CAD build for the part. Positions are in the model's coordinates, mm. A direction names the side the tool comes from. Give positions to 0.01 mm unless a question says otherwise; leave off trailing zeros. Loops run counter-clockwise (first coordinate to the right, second up) from the corner with the lowest first, then second, coordinate; pieces in that order, holes last. Notation, with made-up numbers: M -34.75,76 L -26.75,76 A25 cw -26.75,115 Z; hole C 51.25,25 d4. An arc over 180 degrees is marked long. One line per question, with ' | ' between items.
```python
from build123d import *

# Parameters (mm, degrees)
BOSS_EXTRUDE1_DEPTH      = 1.5
M3_CLEARANCE_HOLE1_D     = 3.2
M3_CLEARANCE_HOLE1_DEPTH = 3
SKETCH5_R                = 15
CUT_EXTRUDE1_DEPTH       = 1
CUT_EXTRUDE1_DEPTH_BACK  = 4
SKETCH6_R                = 13
BOSS_EXTRUDE2_DEPTH      = 40
M6_CLEARANCE_HOLE1_D     = 6.4
M6_CLEARANCE_HOLE1_DEPTH = 10
SKETCH11_OUTSIDE_W       = 233.632
SKETCH11_OUTSIDE_H       = 233.632
CUT_EXTRUDE2_DEPTH       = 40
SKETCH12_W               = 183.089507272
SKETCH12_H               = 5.144734847
CUT_EXTRUDE4_DEPTH       = 91
CUT_EXTRUDE4_DEPTH_BACK  = 91


with BuildPart() as part:
    # Sketch1 → Boss-Extrude1 (new body, symmetric)
    with BuildSketch(Plane(origin=(0, 0, 0), x_dir=(1, 0, 0), z_dir=(0, 1, 0))):
        with BuildLine():
            Line((50, 10), (84, 10))
            ThreePointArc((84, 10), (88.242640687, 8.242640687), (90, 4))
            Line((90, 4), (90, -4))
            ThreePointArc((90, -4), (88.242640687, -8.242640687), (84, -10))
            Line((84, -10), (50, -10))
            ThreePointArc((50, -10), (21.715728753, -21.715728753), (10, -50))
            Line((10, -50), (10, -84))
            ThreePointArc((10, -84), (8.242640687, -88.242640687), (4, -90))
            Line((4, -90), (-4, -90))
            ThreePointArc((-4, -90), (-8.242640687, -88.242640687), (-10, -84))
            Line((-10, -84), (-10, -50))
            ThreePointArc((-10, -50), (-21.715728753, -21.715728753), (-50, -10))
            Line((-50, -10), (-84, -10))
            ThreePointArc((-84, -10), (-88.242640687, -8.242640687), (-90, -4))
            Line((-90, -4), (-90, 4))
            ThreePointArc((-90, 4), (-88.242640687, 8.242640687), (-84, 10))
            Line((-84, 10), (-50, 10))
            ThreePointArc((-50, 10), (-21.715728753, 21.715728753), (-10, 50))
            Line((-10, 50), (-10, 84))
            ThreePointArc((-10, 84), (-8.242640687, 88.242640687), (-4, 90))
            Line((-4, 90), (4, 90))
            ThreePointArc((4, 90), (8.242640687, 88.242640687), (10, 84))
            Line((10, 84), (10, 50))
            ThreePointArc((10, 50), (21.715728753, 21.715728753), (50, 10))
        make_face()
    extrude(amount=BOSS_EXTRUDE1_DEPTH, both=True)

    # M3 Clearance Hole1
    with Locations(Plane(origin=(0, 1.5, 0), x_dir=(1, 0, 0), z_dir=(0, 1, 0))):
        with Locations((-84, 4), (-84, -4), (-4, 84), (4, 84), (84, 4), (84, -4), (4, -84), (-4, -84), (-39, 4), (-39, -4), (39, 4), (39, -4), (4, -39), (-4, -39), (-4, 39), (4, 39)):
            Hole(M3_CLEARANCE_HOLE1_D / 2, depth=M3_CLEARANCE_HOLE1_DEPTH)

    # Sketch5 → Cut-Extrude1 (cut, two sides)
    with BuildSketch(Plane(origin=(0, 1.5, 0), x_dir=(1, 0, 0), z_dir=(0, 1, 0))) as cut_extrude1_sk:
        Circle(SKETCH5_R)
    extrude(amount=CUT_EXTRUDE1_DEPTH, mode=Mode.SUBTRACT)
    extrude(cut_extrude1_sk.sketch, amount=-CUT_EXTRUDE1_DEPTH_BACK, mode=Mode.SUBTRACT)

    # Sketch6 → Boss-Extrude2 (add)
    with BuildSketch(Plane.XZ.offset(1.5)):
        with BuildLine():
            Line((-15.762553167, 8.691485355), (-25.473103505, 18.402035693))
            Line((-25.473103505, 18.402035693), (-18.402035693, 25.473103505))
            Line((-18.402035693, 25.473103505), (-8.691485355, 15.762553167))
            ThreePointArc((-8.691485355, 15.762553167), (12.727922061, 12.727922061), (15.762553167, -8.691485355))
            Line((15.762553167, -8.691485355), (25.473103505, -18.402035693))
            Line((25.473103505, -18.402035693), (18.402035693, -25.473103505))
            Line((18.402035693, -25.473103505), (8.691485355, -15.762553167))
            ThreePointArc((8.691485355, -15.762553167), (-12.727922061, -12.727922061), (-15.762553167, 8.691485355))
        make_face()
        Circle(SKETCH6_R, mode=Mode.SUBTRACT)
    extrude(amount=BOSS_EXTRUDE2_DEPTH)

    # M6 Clearance Hole1
    with Locations(Plane(origin=(3.535533906, 0, 3.535533906), x_dir=(0.707106781, 0, -0.707106781), z_dir=(0.707106781, 0, 0.707106781))):
        with Locations((-24.158012459, -11.5), (-24.158012459, -31.5), (24.158012459, -11.5), (24.158012459, -31.5)):
            Hole(M6_CLEARANCE_HOLE1_D / 2, depth=M6_CLEARANCE_HOLE1_DEPTH)

    # Sketch11 outside → Cut-Extrude2 (cut)
    with BuildSketch(Plane.XZ.offset(41.5)):
        Rectangle(SKETCH11_OUTSIDE_W, SKETCH11_OUTSIDE_H)
        with BuildLine():
            Line((-21.937569599, 21.937569599), (21.937569599, -21.937569599))
            Line((21.937569599, -21.937569599), (18.402035693, -25.473103505))
            Line((18.402035693, -25.473103505), (8.691485355, -15.762553167))
            ThreePointArc((8.691485355, -15.762553167), (-12.727922061, -12.727922061), (-15.762553167, 8.691485355))
            Line((-15.762553167, 8.691485355), (-25.473103505, 18.402035693))
            Line((-25.473103505, 18.402035693), (-21.937569599, 21.937569599))
        make_face(mode=Mode.SUBTRACT)
    extrude(amount=-CUT_EXTRUDE2_DEPTH, mode=Mode.SUBTRACT)

    # Sketch12 → Cut-Extrude4 (cut, two sides)
    with BuildSketch(Plane(origin=(0, 0, 0), x_dir=(0, 0, -1), z_dir=(1, 0, 0))) as cut_extrude4_sk:
        with Locations((-1.544753636, 1.072367424)):
            Rectangle(SKETCH12_W, SKETCH12_H)
    extrude(amount=CUT_EXTRUDE4_DEPTH, mode=Mode.SUBTRACT)
    extrude(cut_extrude4_sk.sketch, amount=-CUT_EXTRUDE4_DEPTH_BACK, mode=Mode.SUBTRACT)


solid = part.part
```
Item 1: Drill centre lines: line 1 along Z through (x, y) = (-11.5, -21); line 2 along Z through (x, y) = (0.5, -27.5); line 3 along Z through (x, y) = (7, -22.5). Where is each one in solid material? Low to high. Write a range as [from, to].
Conclusion:
line 1: [-13.85, -6.06], [6.06, 11.5] | line 2: [-17.99, -12.99] | line 3: [-16.58, -10.95]
Item 2: 3-axis set-ups, long thin cutter, end or side, ignore diameter. For faces 1 (the cylindrical face through (-17.079, -13.447, 13.494)), 2 (the flat face through (13.615, -21.22, -20.686)): which of +Z, -Z, +X, -X, +Y, -Y reach the whole face in a straight line?
Conclusion:
face 1: none | face 2: -Z, +Y, -Y
Item 3: Saw through at C-C on z = 0. Give the cut face in (x, y), and give its area (3 significant figures).
Conclusion:
outline: M -18,-41.5 L -13,-41.5 L -13,-1.5 L -18,-1.5 Z | area: 200 mm²
Item 4: Mould opens along X. For faces 3 (the cylindrical face through (15.584, -28.327, -19.169)), 4 (the flat face through (-10, -1.5, -9)), 5 (the cylindrical face through (-12.496, -21.22, -12.956)), 6 (the flat face through (-20.55, -21.22, 13.48)) say: pulls with the +X half, pulls with the -X half, needs draft (parallel to the pull), parting line crosses it, or undercut.
Conclusion:
face 3: undercut | face 4: needs draft | face 5: undercut | face 6: pulls with the -X half
Item 5: Saw through at B-B on x = 0. Give the cut face in (y, z).
Conclusion:
outline: M -41.5,-18 L -1.5,-18 L -1.5,-13 L -41.5,-13 Z
Item 6: Drop flat-ended pins along their axis: P1, Ø6, axis at y = -23.5, z = -8.5, coming from the +X side; P2, Ø4, axis at x = -1, y = -28.5, coming from the -Z side; P3, Ø8, axis at x = 13.5, y = -13.5, coming from the +Z side. Give the stop position or say it passes through.
Conclusion:
P1: x = 11.5 | P2: z = -18 | P3: z = -9.5
